Can you work these out from the drawing? Everything is in mm from the part's minimum corner. A direction names the side the tool comes from. Round coordinates to 2 decimals unless told otherwise and drop trailing zeros. Write each loop counter-clockwise with the first axis right and the second up, starting at its lowest first coordinate (ties: lowest second). Pieces come first, ordered by that corner, then holes. Notation, with made-up numbers: (49.25, 6.5) -> (98.25, 6.5) arc R16 ccw to (98.25, 37.5) -> close; hole circle Ø1 at (84.5, -26.75). An arc over 180 degrees is marked (long way). One line per question, with ' | ' between items. Start each with the question number.
1. For pin 1 Ø2 at (x, y) = (94, 8.5) entering from +Z; pin 2 Ø2.5 at (y, z) = (5, 111) entering from +X; pin 3 Ø10.5 at (x, z) = (25.5, 23.5) entering from +Y (3 decimals), each with a flat end and sliding along its axis, tell me the tip position at first contact or that it passes through.
2. Thinking about a two-plate mould opening in X: for the marked faces 3 and 4, which applies, released by +X, released by -X, zero draft, split by the parting line, or undercut?
3. Imagine slicing it at A-A, the plane y = 4.75. List the corners of the cut face in (x, z) for me.
4. Imagine slicing it at B-B, the plane z = 82. List the corners of the cut face in (x, y) for me (3 decimals).
5. Imagine slicing it at C-C, the plane x = 9. List the corners of the cut face in (y, z) for me (3 decimals).
6. Imagine slicing it at D-D, the plane z = 12.5. List the corners of the cut face in (x, y) for me (3 decimals), and give its area (3 significant figures).
7. If I drill on line 1 along X through (y, z) = (4, 39); line 2 along X through (y, z) = (7.25, 68); line 3 along Z through (x, y) = (49, 5.75), over which ranges is the centre line in solid material (lowest first)? Write a range as [from, to].
8. For the marked faces 1 and 2, which set-ups out of +Z, -Z, +X, -X, +Y, -Y let a thin tool reach every point of the face, with its end or its side?
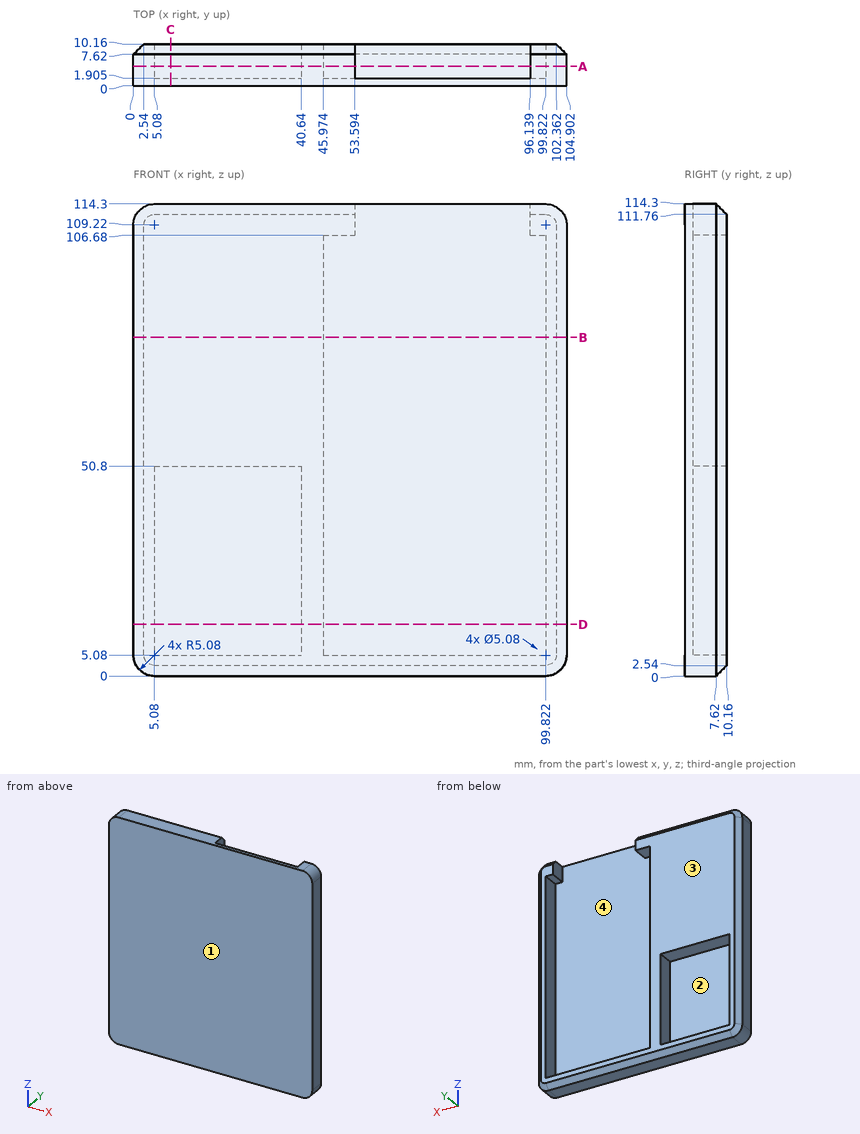
Geometry results:
1) pin 1: stops at z = 5.08 | pin 2: stops at x = 104.87 | pin 3: stops at y = 1.905
2) face 3: zero draft | face 4: undercut
3) outline: (0, 5.08) arc R5.08 ccw to (5.08, 0) -> (99.82, 0) arc R5.08 ccw to (104.9, 5.08) -> (104.9, 109.22) arc R5.08 ccw to (99.82, 114.3) -> (96.14, 114.3) -> (96.14, 106.68) -> (99.82, 106.68) -> (99.82, 5.08) -> (45.97, 5.08) -> (45.97, 106.68) -> (53.59, 106.68) -> (53.59, 114.3) -> (5.08, 114.3) arc R5.08 ccw to (0, 109.22) -> close; hole (5.08, 5.08) -> (40.64, 5.08) -> (40.64, 50.8) -> (5.08, 50.8) -> close
4) outline: (0, 0) -> (104.902, 0) -> (104.902, 7.62) -> (102.362, 10.16) -> (99.822, 10.16) -> (99.822, 1.905) -> (45.974, 1.905) -> (45.974, 10.16) -> (2.54, 10.16) -> (0, 7.62) -> close
5) outline: (0, 0) -> (7.62, 0) -> (10.16, 2.54) -> (10.16, 5.08) -> (1.905, 5.08) -> (1.905, 50.8) -> (10.16, 50.8) -> (10.16, 111.76) -> (7.62, 114.3) -> (0, 114.3) -> close
6) outline: (0, 0) -> (104.902, 0) -> (104.902, 7.62) -> (102.362, 10.16) -> (99.822, 10.16) -> (99.822, 1.905) -> (45.974, 1.905) -> (45.974, 10.16) -> (40.64, 10.16) -> (40.64, 1.905) -> (5.08, 1.905) -> (5.08, 10.16) -> (2.54, 10.16) -> (0, 7.62) -> close | area: 321 mm2
7) line 1: x = [0, 5.08], [40.64, 45.97], [99.82, 104.9] | line 2: x = [0, 45.97], [99.82, 104.9] | line 3: z = [0, 5.08], [106.68, 114.3]
8) face 1: +Z, -Z, +X, -X, -Y | face 2: +Y
